Model file for the job. Use its own axes, mm. A direction names the side the tool comes from. Coordinates: 2 decimals unless noted, no trailing zeros. Order: outer loops, then holes, each group sorted by start corner. A loop starts at its lowest first (then second) coordinate and runs counter-clockwise, first axis right, second up. Notation, with made-up numbers: (40, 88.5) -> (57, 88.5) arc R21 ccw to (57, 110.5) -> close; hole circle Ø4 at (-22, 84). An arc over 180 degrees is marked (long way). Use CSV: the item, a comma, the result in double quotes. Start each with the question number.
(1) Cut at A-A on z = 15.5. Write the cut outline in (x, y).
(2) Tool access for faces 1 (the flat face through (0, 0, -3)), 2 (the flat face through (2.321, -1, 18)): list every direction of +Z, -Z, +X, -X, +Y, -Y with a clear straight run to the whole face (end or side of a thin tool).
(3) Pin check, flat tip, straight feed: pin 1 Ø4 at (x, z) = (27, -2) entering from -Y. Stop position of the tip, or through.
(4) Cut at D-D on x = 0. Write the cut outline in (y, z), plus the area to 3 significant figures.
(5) Pull direction X, two halves, no side cores. Call faces 3 (the flat face through (-34.671, -1, 15)), 4 (the flat face through (-1, -1, -38.1)): pulls with the +X half, pulls with the -X half, needs draft (parallel to the pull), parting line crosses it, or undercut.
(6) Cut at C-C on z = 0. Write the cut outline in (x, y).
(7) Cut at B-B on x = 16. Write the cut outline in (y, z).
(8) Probe L1, parallel to X at y = -2.1, z = 22; L2, parallel to Z at x = -3, y = -0.8; L3, parallel to Z at x = 30, y = -1.15. List the from-to ranges inside material, lowest first.
```python
from build123d import *

# Parameters (mm, degrees)
F0_W     = 76.2
F0_H     = 76.2
F0_W_2   = 6.35
F0_H_2   = 6.35
F1_DEPTH = 3
F2_D     = 2


with BuildPart() as f1:
    # F0 (on Front) → F1 (new body)
    with BuildSketch(Plane.XZ):
        Rectangle(F0_W, F0_H)
        Polygon((-34.671, -34.671), (-34.671, -28.321), (-34.671, -1.671), (-28.321, -1.671), (-2.321, -1.671), (-2.321, -34.671), (-28.321, -34.671), align=None, mode=Mode.SUBTRACT)
        Polygon((34.671, -1.671), (34.671, -28.321), (34.671, -34.671), (28.321, -34.671), (2.321, -34.671), (2.321, -1.671), (28.321, -1.671), align=None, mode=Mode.SUBTRACT)
        Polygon((-34.671, 34.671), (-28.321, 34.671), (-2.321, 34.671), (-2.321, 1.671), (-28.321, 1.671), (-34.671, 1.671), (-34.671, 28.321), align=None, mode=Mode.SUBTRACT)
        Polygon((28.321, 34.671), (34.671, 34.671), (34.671, 28.321), (34.671, 1.671), (28.321, 1.671), (2.321, 1.671), (2.321, 34.671), align=None, mode=Mode.SUBTRACT)
        with Locations((-31.496, 31.496)):
            Rectangle(F0_W_2, F0_H_2)
        with Locations((31.496, 31.496)):
            Rectangle(F0_W_2, F0_H_2)
        with Locations((-31.496, -31.496)):
            Rectangle(F0_W_2, F0_H_2)
        with Locations((31.496, -31.496)):
            Rectangle(F0_W_2, F0_H_2)
    extrude(amount=F1_DEPTH)

    # F2 (through all)
    with Locations(Plane(origin=(0, 0, 0), x_dir=(1, 0, 0), z_dir=(0, 1, 0))):
        with Locations((-31.496, 31.496), (31.496, 31.496), (0, 0), (-31.496, -31.496), (31.496, -31.496)):
            Hole(F2_D / 2)


solid = f1.part
```
Outcome:
1,outline,"(-38.1, -3) -> (-34.67, -3) -> (-34.67, 0) -> (-38.1, 0) -> close; (-2.32, -3) -> (2.32, -3) -> (2.32, 0) -> (-2.32, 0) -> close; (34.67, -3) -> (38.1, -3) -> (38.1, 0) -> (34.67, 0) -> close"
2,face 1,"+Z, -Z, +X, -X, +Y"
2,face 2,"+Y, -Y"
3,pin 1,"y = -3"
4,outline,"(-3, -38.1) -> (0, -38.1) -> (0, -1) -> (-3, -1) -> close; (-3, 1) -> (0, 1) -> (0, 38.1) -> (-3, 38.1) -> close"
4,area,"223 mm2"
5,face 3,"undercut"
5,face 4,"needs draft"
6,outline,"(-38.1, -3) -> (-1, -3) -> (-1, 0) -> (-38.1, 0) -> close; (1, -3) -> (38.1, -3) -> (38.1, 0) -> (1, 0) -> close"
7,outline,"(-3, -38.1) -> (0, -38.1) -> (0, -34.67) -> (-3, -34.67) -> close; (-3, -1.67) -> (0, -1.67) -> (0, 1.67) -> (-3, 1.67) -> close; (-3, 34.67) -> (0, 34.67) -> (0, 38.1) -> (-3, 38.1) -> close"
8,L1,"-38.1 to -34.67, -2.32 to 2.32, 34.67 to 38.1"
8,L2,"-38.1 to -34.67, -1.67 to 1.67, 34.67 to 38.1"
8,L3,"-38.1 to -28.32, -1.67 to 1.67, 28.32 to 38.1"
